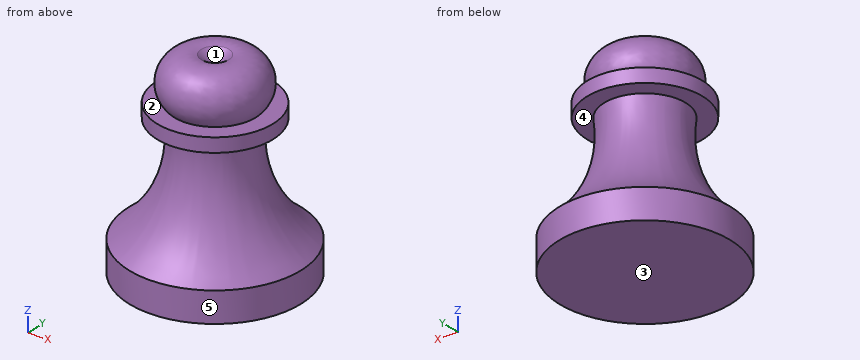
```python
from build123d import *


with BuildPart() as f1:
    # F0 (on Right) → F1 (revolve)
    with BuildSketch(Plane.YZ):
        with BuildLine():
            Line((-29.843854, 0), (0, 0))
            Line((0, 0), (0, 64.164288))
            Line((0, 64.164288), (-4.849625, 67.894772))
            ThreePointArc((-4.849625, 67.894772), (-15.301636, 64.051876), (-14.175827, 52.972846))
            Line((-14.175827, 52.972846), (-20.144602, 52.972846))
            Line((-20.144602, 52.972846), (-20.144602, 48.123218))
            Line((-20.144602, 48.123218), (-14.175827, 48.123218))
            ThreePointArc((-14.175827, 48.123218), (-16.847024, 27.13737), (-29.843854, 10.445351))
            Line((-29.843854, 10.445351), (-29.843854, 0))
        make_face()
    revolve(axis=Axis((0, 0, 32.082144), (0, 0, 1)))


solid = f1.part
```
Verification items for the finished model (mm, model axes). Face numbers are marked on the shaded views. A direction names the side the tool comes from. Give positions to 0.01 mm unless a question says otherwise; leave off trailing zeros. Order: outer loops, then holes, each group sorted by start corner. A loop starts at its lowest first (then second) coordinate and runs counter-clockwise, first axis right, second up. Notation, with made-up numbers: M -6.75,66.25 L 43.25,66.25 A22 cw 43.25,89.25 Z; hole C -30,81.25 d9. An arc over 180 degrees is marked long. Answer in a Markdown table with one row per item. Add a question column.
Item 1: Mould release check, pull along Z, two halves, no side actions. Record for the marked faces 3, 4 and 5: released by +Z, released by -Z, zero draft, split by the parting line, or undercut.
Item 2: Section check A-A, the plane z = 14. Enter the section's corners in (x, y).
Item 3: Scan lines: probe 1 along Z at (x, y) = (11, 13.5); probe 2 along Y at (x, z) = (5, 56.5); probe 3 along X at (y, z) = (-1, 17.5). Record each from-to range of solid material in increasing order. Write a range as from..to.
Item 4: Gauge pin test, flat ends, axial feed: pin 1 (10 mm diameter, centred on y = 16, z = 28, fed in from -X); pin 2 (6 mm diameter, centred on x = -4.5, z = 47, fed in from -Y); pin 3 (8 mm diameter, centred on x = 21.5, y = -20, fed in from +Z). Record the tip position at first contact, or that the pin passes through.
Item 5: Tool access check on the marked faces 1 and 2. Record the directions out of +Z, -Z, +X, -X, +Y, -Y that give a thin tool (end or side, any length) a straight path to the whole face; none if there is none.
Filled sheet:
| question | item | result |
|---|---|---|
| 1 | face 3 | released by -Z |
| 1 | face 4 | undercut |
| 1 | face 5 | zero draft |
| 2 | outline | C 0,0 d51.42 |
| 3 | probe 1 | z = 0..25.84, 48.12..52.97 |
| 3 | probe 2 | y = -15.47..15.47 |
| 3 | probe 3 | x = -22.53..22.53 |
| 4 | pin 1 | stops at x = -13.16 |
| 4 | pin 2 | stops at y = -20.07 |
| 4 | pin 3 | stops at z = 14.34 |
| 5 | face 1 | +Z |
| 5 | face 2 | none |
